```python
from build123d import *

# Parameters (mm, degrees)
SKETCH1_W           = 306.04968
SKETCH1_H           = 38.1
BOSS_EXTRUDE1_DEPTH = 266.7
SKETCH2_W           = 256.243215467
SKETCH2_H           = 152.4
CUT_EXTRUDE1_DEPTH  = 310.83399048


with BuildPart() as part:
    # Sketch1 → Boss-Extrude1 (new body)
    with BuildSketch(Plane.XY):
        Rectangle(SKETCH1_W, SKETCH1_H)
    extrude(amount=-BOSS_EXTRUDE1_DEPTH)

    # Sketch2 → Cut-Extrude1 (cut, through all)
    with BuildSketch(Plane.XZ.offset(19.05)):
        with Locations((-0.496767734, -135.091612863)):
            Rectangle(SKETCH2_W, SKETCH2_H)
    extrude(amount=-CUT_EXTRUDE1_DEPTH, mode=Mode.SUBTRACT)


solid = part.part
```
Verification items for the finished model (mm, model axes). A direction names the side the tool comes from. Coordinates: 2 decimals unless noted, no trailing zeros. Loops run counter-clockwise (first coordinate to the right, second up) from the corner with the lowest first, then second, coordinate; pieces in that order, holes last. Notation, with made-up numbers: (-3, -34) - (44, -34) arc R16 cw to (44, -4) - close; hole circle Ø6 at (-24.75, -21). An arc over 180 degrees is marked (long way). Answer as a JSON object with one key per item and string values.
(1) Scan lines: line 1 along Z through (x, y) = (110, 12.5); line 2 along X through (y, z) = (-15, -74.5). Record each from-to range of solid material in increasing order.
Response:
{"line 1": "z = -266.7 to -211.29, -58.89 to 0", "line 2": "x = -153.02 to -128.62, 127.62 to 153.02"}
(2) Go/stop test with a flat-tipped pin: pin 1 Ø12 at (x, z) = (-33, -205) entering from -Y. Record where the tip stops, or that it passes through.
Response:
{"pin 1": "passes through"}
(3) Access from +Z, -Z, +X, -X, +Y, -Y to the whole of each face (thin tool, end or side, straight path). Record for faces 1 (the flat face through (-2, -19.05, -43)), 2 (the flat face through (-2, 0, -211.292)).
Response:
{"face 1": "+Z, -Z, +X, -X, -Y", "face 2": "+Y, -Y"}
(4) Cross-section at A-A, the plane z = -172.5. Record the boundary of the cut face in (x, y), then the cut area to 3 significant figures.
Response:
{"outline": "(-153.02, -19.05) - (-128.62, -19.05) - (-128.62, 19.05) - (-153.02, 19.05) - close; (127.62, -19.05) - (153.02, -19.05) - (153.02, 19.05) - (127.62, 19.05) - close", "area": "1,900 mm²"}
(5) Mould release check, pull along Z, two halves, no side actions. Record for faces 3 (the flat face through (-2, 0, -266.7)), 4 (the flat face through (-2, 0, 0)), 5 (the flat face through (-128.618, 0, -136)): pulls with the +Z half, pulls with the -Z half, needs draft (parallel to the pull), parting line crosses it, or undercut.
Response:
{"face 3": "pulls with the -Z half", "face 4": "pulls with the +Z half", "face 5": "undercut"}
(6) Cross-section at C-C, the plane y = -7. Record the boundary of the cut face in (x, z).
Response:
{"outline": "(-153.02, -266.7) - (153.02, -266.7) - (153.02, 0) - (-153.02, 0) - close; hole (-128.62, -211.29) - (127.62, -211.29) - (127.62, -58.89) - (-128.62, -58.89) - close"}
(7) Cross-section at B-B, the plane x = 104.5. Record the boundary of the cut face in (y, z), then the cut area to 3 significant figures.
Response:
{"outline": "(-19.05, -266.7) - (19.05, -266.7) - (19.05, -211.29) - (-19.05, -211.29) - close; (-19.05, -58.89) - (19.05, -58.89) - (19.05, 0) - (-19.05, 0) - close", "area": "4,350 mm²"}
